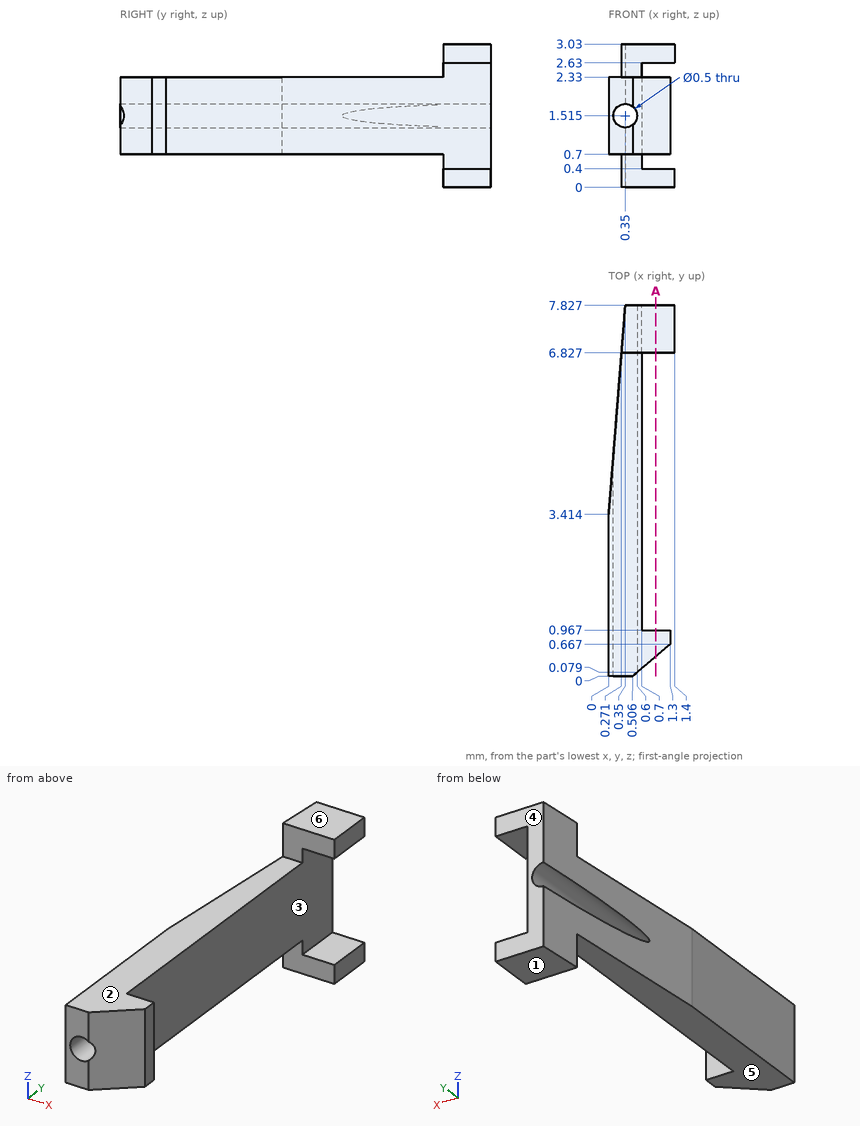
Print and shaded views of the part. All mm, measured from the part's lowest x, y and z. A direction names the side the tool comes from. Give positions to 0.01 mm unless a question says otherwise; leave off trailing zeros. Use CSV: the item, a comma, the result in double quotes. Start each with the question number.
1) Wall check: line 1 (Z direction, x = 0.35, y = 2.75) (1 decimal); line 2 (Y direction, x = 0.65, z = 0.55); line 3 (X direction, y = 1.75, z = 1.05). Give the ranges that are in metal, low to high.
2) Mould opens along Z. For the marked faces 3, 4, 5 and 6 say: released by +Z, released by -Z, zero draft, split by the parting line, or undercut.
3) Tool access for the marked faces 1 and 2: list every direction of +Z, -Z, +X, -X, +Y, -Y with a clear straight run to the whole face (end or side of a thin tool).
4) Slice it at A-A on x = 1. Give the number of separate pieces and of enclosed holes in the cut face.
5) Flat gauge pins, fed straight in: pin 1 Ø1 at (y, z) = (5, 1) entering from -X; pin 2 Ø0.8 at (x, z) = (0.5, 3) entering from -Y; pin 3 Ø1.5 at (y, z) = (1.5, 0.5) entering from -X; pin 4 Ø0.8 at (x, z) = (1, 0.5) entering from -Y (1 decimal). Where does each tip first touch, or does it go through?
Computed values:
1,line 1,"z = 0.7 to 1.3, 1.8 to 2.3"
1,line 2,"y = 6.83 to 7.83"
1,line 3,"x = 0 to 0.7"
2,face 3,"undercut"
2,face 4,"zero draft"
2,face 5,"released by -Z"
2,face 6,"released by +Z"
3,face 1,"-Z, +X, -X, +Y, -Y"
3,face 2,"+Z, +X, -X, -Y"
4,separate pieces,"3"
4,enclosed holes,"0"
5,pin 1,"stops at x = 0.09"
5,pin 2,"stops at y = 6.83"
5,pin 3,"stops at x = 0"
5,pin 4,"stops at y = 0.1"
